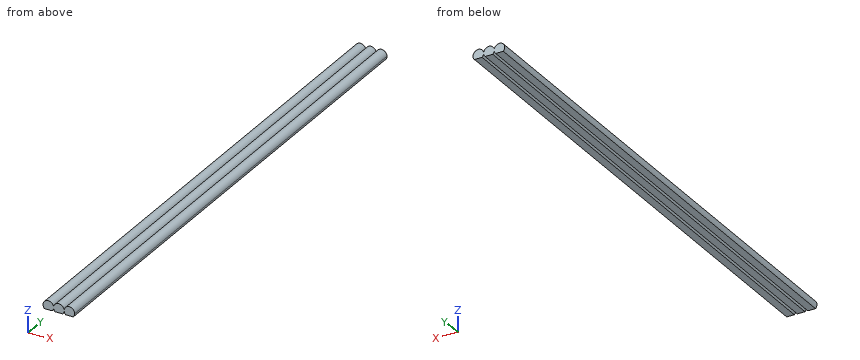
```python
from build123d import *

# Parameters (mm, degrees)
F1_DEPTH = 317.5


with BuildPart() as f1:
    # F0 (on Front) → F1 (new body)
    with BuildSketch(Plane.XZ):
        with BuildLine():
            ThreePointArc((3.0642884432, 0.8311205311), (-1.5592869758, 2.7657275945), (-2.2972373281, -2.1916490728))
            Line((-2.2972373281, -2.1916490728), (2.2972373281, -2.1916490728))
            ThreePointArc((2.2972373281, -2.1916490728), (2.7781759552, -1.5369981658), (3.0772573724, -0.7817365695))
            Line((3.0772573724, -0.7817365695), (2.3432357702, -0.7817365695))
            Line((2.3432357702, -0.7817365695), (2.3432357702, 0.8311205311))
            Line((2.3432357702, 0.8311205311), (3.0642884432, 0.8311205311))
        make_face()
        with BuildLine():
            ThreePointArc((3.2857115568, 0.8311205311), (3.2027995927, 0.4192309584), (3.175, 0))
            ThreePointArc((3.175, 0), (3.1995304193, -0.3939116923), (3.2727426276, -0.7817365695))
            Line((3.2727426276, -0.7817365695), (4.0206070989, -0.7817365695))
            Line((4.0206070989, -0.7817365695), (4.0206070989, 0.8311205311))
            Line((4.0206070989, 0.8311205311), (3.2857115568, 0.8311205311))
        make_face()
        with BuildLine():
            ThreePointArc((3.175, 0), (3.1472004073, 0.4192309584), (3.0642884432, 0.8311205311))
            Line((3.0642884432, 0.8311205311), (2.3432357702, 0.8311205311))
            Line((2.3432357702, 0.8311205311), (2.3432357702, -0.7817365695))
            Line((2.3432357702, -0.7817365695), (3.0772573724, -0.7817365695))
            ThreePointArc((3.0772573724, -0.7817365695), (3.1504695807, -0.3939116923), (3.175, 0))
        make_face()
        with BuildLine():
            Line((3.2857115568, 0.8311205311), (3.0642884432, 0.8311205311))
            ThreePointArc((3.0642884432, 0.8311205311), (3.1472004073, 0.4192309584), (3.175, 0))
            ThreePointArc((3.175, 0), (3.2027995927, 0.4192309584), (3.2857115568, 0.8311205311))
        make_face()
        with BuildLine():
            ThreePointArc((3.175, 0), (3.1504695807, -0.3939116923), (3.0772573724, -0.7817365695))
            Line((3.0772573724, -0.7817365695), (3.2727426276, -0.7817365695))
            ThreePointArc((3.2727426276, -0.7817365695), (3.1995304193, -0.3939116923), (3.175, 0))
        make_face()
        with BuildLine():
            ThreePointArc((3.2727426276, -0.7817365695), (3.5718240448, -1.5369981658), (4.0527626719, -2.1916490728))
            Line((4.0527626719, -2.1916490728), (8.6472373281, -2.1916490728))
            ThreePointArc((8.6472373281, -2.1916490728), (9.1697839759, -1.4592612272), (9.4659095878, -0.6096986472))
            Line((9.4659095878, -0.6096986472), (9.0097114444, -0.6096986472))
            Line((9.0097114444, -0.6096986472), (9.0097114444, 0.6375776138))
            Line((9.0097114444, 0.6375776138), (9.4603247075, 0.6375776138))
            ThreePointArc((9.4603247075, 0.6375776138), (6.4494713507, 3.1734414207), (3.2857115568, 0.8311205311))
            Line((3.2857115568, 0.8311205311), (4.0206070989, 0.8311205311))
            Line((4.0206070989, 0.8311205311), (4.0206070989, -0.7817365695))
            Line((4.0206070989, -0.7817365695), (3.2727426276, -0.7817365695))
        make_face()
        with BuildLine():
            ThreePointArc((9.525, 0), (9.5087897957, 0.3204247599), (9.4603247075, 0.6375776138))
            Line((9.4603247075, 0.6375776138), (9.0097114444, 0.6375776138))
            Line((9.0097114444, 0.6375776138), (9.0097114444, -0.6096986472))
            Line((9.0097114444, -0.6096986472), (9.4659095878, -0.6096986472))
            ThreePointArc((9.4659095878, -0.6096986472), (9.5101928692, -0.3062776996), (9.525, 0))
        make_face()
        with BuildLine():
            ThreePointArc((9.5840904122, -0.6096986472), (9.8802160241, -1.4592612272), (10.4027626719, -2.1916490728))
            Line((10.4027626719, -2.1916490728), (14.9972373281, -2.1916490728))
            ThreePointArc((14.9972373281, -2.1916490728), (15.6474016961, -1.1804440866), (15.875, 0))
            ThreePointArc((15.875, 0), (13.0204247599, 3.1587897957), (9.5896752925, 0.6375776138))
            Line((9.5896752925, 0.6375776138), (10.278493166, 0.6375776138))
            Line((10.278493166, 0.6375776138), (10.278493166, -0.6096986472))
            Line((10.278493166, -0.6096986472), (9.5840904122, -0.6096986472))
        make_face()
        with BuildLine():
            ThreePointArc((9.5896752925, 0.6375776138), (9.5412102043, 0.3204247599), (9.525, 0))
            ThreePointArc((9.525, 0), (9.5398071308, -0.3062776996), (9.5840904122, -0.6096986472))
            Line((9.5840904122, -0.6096986472), (10.278493166, -0.6096986472))
            Line((10.278493166, -0.6096986472), (10.278493166, 0.6375776138))
            Line((10.278493166, 0.6375776138), (9.5896752925, 0.6375776138))
        make_face()
        with BuildLine():
            Line((9.5896752925, 0.6375776138), (9.4603247075, 0.6375776138))
            ThreePointArc((9.4603247075, 0.6375776138), (9.5087897957, 0.3204247599), (9.525, 0))
            ThreePointArc((9.525, 0), (9.5412102043, 0.3204247599), (9.5896752925, 0.6375776138))
        make_face()
        with BuildLine():
            ThreePointArc((9.525, 0), (9.5101928692, -0.3062776996), (9.4659095878, -0.6096986472))
            Line((9.4659095878, -0.6096986472), (9.5840904122, -0.6096986472))
            ThreePointArc((9.5840904122, -0.6096986472), (9.5398071308, -0.3062776996), (9.525, 0))
        make_face()
    extrude(amount=F1_DEPTH)


solid = f1.part
```
Could you check a few things on this model? Use its own coordinates, in mm. Coordinates: 2 decimals unless noted, no trailing zeros. Write each loop counter-clockwise with the first axis right and the second up, starting at its lowest first coordinate (ties: lowest second). Pieces come first, ordered by that corner, then holes. Notation, with made-up numbers: (42.25, -2.5) -> (66.25, -2.5) arc R34 ccw to (66.25, 31.5) -> close; hole circle Ø11 at (59, 72). An arc over 180 degrees is marked (long way). One line per question, with ' | ' between items. Start each with the question number.
1. Please list where these lines run through material, in increasing order: line 1 along X through (y, z) = (-62, -1.45); line 2 along X through (y, z) = (-245, 2.35); line 3 along Z through (x, y) = (7, -304).
2. If we section it at A-A (y = -24): Please give me the cut outline in (x, z) (3 decimals), and give its area (3 significant figures).
3. Will these pins go through, and if not, where does the flat tip stop? P1, Ø1, axis at y = -88.5, z = 2.5, coming from the +X side; P2, Ø2, axis at x = 4.5, y = -104.5, coming from the +Z side.
Return value:
1) line 1: x = -2.82 to 2.82, 3.53 to 9.17, 9.88 to 15.52 | line 2: x = -2.13 to 2.13, 4.22 to 8.48, 10.57 to 14.83 | line 3: z = -2.19 to 3.11
2) outline: (-2.297, -2.192) -> (2.297, -2.192) arc R3.175 ccw to (3.077, -0.782) -> (3.273, -0.782) arc R3.175 ccw to (4.053, -2.192) -> (8.647, -2.192) arc R3.175 ccw to (9.466, -0.61) -> (9.584, -0.61) arc R3.175 ccw to (10.403, -2.192) -> (14.997, -2.192) arc R3.175 ccw (long way) to (9.59, 0.638) -> (9.46, 0.638) arc R3.175 ccw to (3.286, 0.831) -> (3.064, 0.831) arc R3.175 ccw (long way) to start | area: 85.8 mm²
3) P1: stops at x = 15.17 | P2: stops at z = 3.06
